For this review, take the finished solid that the model builds, in its own axes (mm). Face numbers are marked on the shaded views. A direction names the side the tool comes from. Give positions to 0.01 mm unless a question says otherwise; leave off trailing zeros. Loops run counter-clockwise (first coordinate to the right, second up) from the corner with the lowest first, then second, coordinate; pieces in that order, holes last.
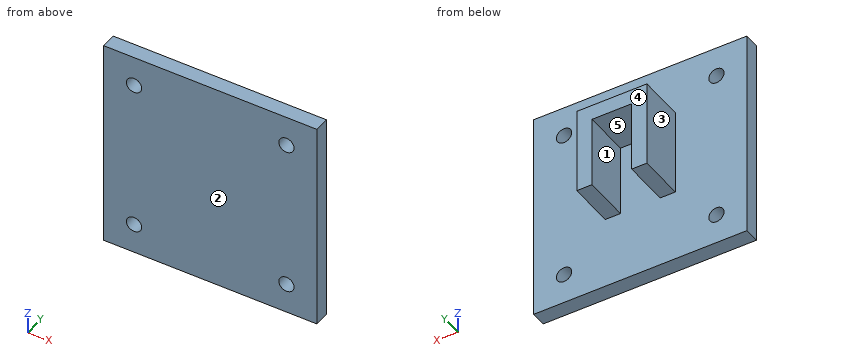
```python
from build123d import *

# Parameters (mm, degrees)
SKETCH1_W           = 70
SKETCH1_H           = 70
BOSS_EXTRUDE1_DEPTH = 5
SKETCH2_R           = 2.5
CUT_EXTRUDE1_DEPTH  = 5
SKETCH3_R           = 2.5
CUT_EXTRUDE2_DEPTH  = 5
SKETCH4_R           = 2.5
CUT_EXTRUDE3_DEPTH  = 5
SKETCH5_R           = 2.5
CUT_EXTRUDE4_DEPTH  = 5
SKETCH6_W           = 23
SKETCH6_H           = 35
BOSS_EXTRUDE2_DEPTH = 15
SKETCH7_W           = 13
SKETCH7_H           = 30
CUT_EXTRUDE5_DEPTH  = 15
SKETCH8_W           = 5
SKETCH8_H           = 6.5
CUT_EXTRUDE6_DEPTH  = 15
SKETCH9_W           = 5
SKETCH9_H           = 6.5
CUT_EXTRUDE7_DEPTH  = 15


with BuildPart() as part:
    # Sketch1 → Boss-Extrude1 (new body)
    with BuildSketch(Plane(origin=(0, 0, 0), x_dir=(1, 0, 0), z_dir=(0, 1, 0))):
        Rectangle(SKETCH1_W, SKETCH1_H)
    extrude(amount=BOSS_EXTRUDE1_DEPTH)

    # Sketch2 → Cut-Extrude1 (cut)
    with BuildSketch(Plane(origin=(0, 5, 0), x_dir=(1, 0, 0), z_dir=(0, 1, 0))):
        with Locations(Location((-25, 25, 0), (0, 0, 270))):
            Circle(SKETCH2_R)
    extrude(amount=-CUT_EXTRUDE1_DEPTH, mode=Mode.SUBTRACT)

    # Sketch3 → Cut-Extrude2 (cut)
    with BuildSketch(Plane(origin=(0, 5, 0), x_dir=(1, 0, 0), z_dir=(0, 1, 0))):
        with Locations(Location((25, 25, 0), (0, 0, 270))):
            Circle(SKETCH3_R)
    extrude(amount=-CUT_EXTRUDE2_DEPTH, mode=Mode.SUBTRACT)

    # Sketch4 → Cut-Extrude3 (cut)
    with BuildSketch(Plane(origin=(0, 5, 0), x_dir=(1, 0, 0), z_dir=(0, 1, 0))):
        with Locations(Location((-25, -25, 0), (0, 0, 270))):
            Circle(SKETCH4_R)
    extrude(amount=-CUT_EXTRUDE3_DEPTH, mode=Mode.SUBTRACT)

    # Sketch5 → Cut-Extrude4 (cut)
    with BuildSketch(Plane(origin=(0, 5, 0), x_dir=(1, 0, 0), z_dir=(0, 1, 0))):
        with Locations(Location((25, -25, 0), (0, 0, 270))):
            Circle(SKETCH5_R)
    extrude(amount=-CUT_EXTRUDE4_DEPTH, mode=Mode.SUBTRACT)

    # Sketch6 → Boss-Extrude2 (add)
    with BuildSketch(Plane(origin=(0, 5, 0), x_dir=(1, 0, 0), z_dir=(0, 1, 0))):
        Rectangle(SKETCH6_W, SKETCH6_H)
    extrude(amount=BOSS_EXTRUDE2_DEPTH)

    # Sketch7 → Cut-Extrude5 (cut)
    with BuildSketch(Plane(origin=(0, 20, 0), x_dir=(1, 0, 0), z_dir=(0, 1, 0))):
        with Locations((0, 2.5)):
            Rectangle(SKETCH7_W, SKETCH7_H)
    extrude(amount=-CUT_EXTRUDE5_DEPTH, mode=Mode.SUBTRACT)

    # Sketch8 → Cut-Extrude6 (cut)
    with BuildSketch(Plane(origin=(0, 20, 0), x_dir=(1, 0, 0), z_dir=(0, 1, 0))):
        with Locations((-9, 14.25)):
            Rectangle(SKETCH8_W, SKETCH8_H)
    extrude(amount=-CUT_EXTRUDE6_DEPTH, mode=Mode.SUBTRACT)

    # Sketch9 → Cut-Extrude7 (cut)
    with BuildSketch(Plane(origin=(0, 20, 0), x_dir=(1, 0, 0), z_dir=(0, 1, 0))):
        with Locations((9, 14.25)):
            Rectangle(SKETCH9_W, SKETCH9_H)
    extrude(amount=-CUT_EXTRUDE7_DEPTH, mode=Mode.SUBTRACT)


solid = part.part
```
Q1. Consider section A-A on x = 25. Give the boundary of the cut face in (y, z).
Answers:
outline: (0, -35) - (5, -35) - (5, -27.5) - (0, -27.5) - close; (0, -22.5) - (5, -22.5) - (5, 22.5) - (0, 22.5) - close; (0, 27.5) - (5, 27.5) - (5, 35) - (0, 35) - close
Q2. Consider section D-D on y = 11. Give the boundary of the cut face in (x, z), plus the area to 3 significant figures.
Answers:
outline: (-11.5, -11) - (-6.5, -11) - (-6.5, 12.5) - (6.5, 12.5) - (6.5, -11) - (11.5, -11) - (11.5, 17.5) - (-11.5, 17.5) - close
area: 350 mm2
Q3. Mouldability with a two-part tool opening along X and no side actions: class the marked faces 3, 4 and 5 as +X half, -X half, draft (parallel to the pull), parting line (faces both ways), or undercut.
Answers:
face 3: -X half
face 4: draft
face 5: undercut
Q4. For probe 1 along X at (y, z) = (2.6, 25); probe 2 along X at (y, z) = (11.5, 11); probe 3 along Y at (x, z) = (-20, 27), list the stretches that pass through material, from the lowest coordinate up.
Answers:
probe 1: x = -35 to -27.5, -22.5 to 22.5, 27.5 to 35
probe 2: x = -11.5 to -6.5, 6.5 to 11.5
probe 3: y = 0 to 5
Q5. Consider section B-B on y = 1.75. Give the boundary of the cut face in (x, z), plus the area to 3 significant figures.
Answers:
outline: (-35, -35) - (35, -35) - (35, 35) - (-35, 35) - close; hole circle Ø5 at (-25, -25); hole circle Ø5 at (-25, 25); hole circle Ø5 at (25, -25); hole circle Ø5 at (25, 25)
area: 4,820 mm2
Q6. Consider section C-C on z = 25. Give the boundary of the cut face in (x, y).
Answers:
outline: (-35, 0) - (-27.5, 0) - (-27.5, 5) - (-35, 5) - close; (-22.5, 0) - (22.5, 0) - (22.5, 5) - (-22.5, 5) - close; (27.5, 0) - (35, 0) - (35, 5) - (27.5, 5) - close
Q7. Machinability: for the marked faces 1 and 2, which of the approach directions +Z, -Z, +X, -X, +Y, -Y give a long, thin tool a straight path to every point of the face, cutting with its end or side? Answer none if there is none.
Answers:
face 1: -Z, +Y
face 2: +Z, -Z, +X, -X, -Y
Q8. For pin 1 Ø10.5 at (x, y) = (0.5, 14.5) entering from -Z; pin 2 Ø12 at (y, z) = (12.5, 5) entering from -X; pin 3 Ø2 at (x, z) = (-3.5, -14.5) entering from +Y, all flat-tipped, find the tip position at first contact; note any pin that passes through.
Answers:
pin 1: stops at z = 12.5
pin 2: stops at x = -11.5
pin 3: stops at y = 5
